from build123d import *

# Parameters (mm, degrees)
SKETCH1_W           = 203.2
SKETCH1_H           = 63.5
BOSS_EXTRUDE1_DEPTH = 3.175
SKETCH2_W           = 15.875
SKETCH2_H           = 6.35
CUT_EXTRUDE1_DEPTH  = 107.634633211
SKETCH3_W           = 19.05
SKETCH3_H           = 6.35
CUT_EXTRUDE2_DEPTH  = 107.634633211
LPATTERN1_COUNT     = 4
LPATTERN1_PITCH     = 38.1
SKETCH4_W           = 6.35
SKETCH4_H           = 19.05
CUT_EXTRUDE3_DEPTH  = 107.634633211


with BuildPart() as part:
    # Sketch1 → Boss-Extrude1 (new, symmetric)
    with BuildSketch(Plane.XY):
        Rectangle(SKETCH1_W, SKETCH1_H)
    extrude(amount=BOSS_EXTRUDE1_DEPTH, both=True)

    # Sketch2 → Cut-Extrude1 (cut, through all)
    with BuildSketch(Plane.XY.offset(3.175)):
        with Locations((-93.6625, 28.575)):
            Rectangle(SKETCH2_W, SKETCH2_H)
    cut_extrude1 = extrude(amount=-CUT_EXTRUDE1_DEPTH, mode=Mode.SUBTRACT)

    # Mirror1: Cut-Extrude1 across plane
    add(cut_extrude1.mirror(Plane(origin=(0, 0, 0), x_dir=(0, 0, 1), z_dir=(1, 0, 0))), mode=Mode.SUBTRACT)

    # Sketch3 → Cut-Extrude2 (cut, through all)
    with BuildSketch(Plane.XY.offset(3.175)):
        with Locations((-57.15, 28.575)):
            Rectangle(SKETCH3_W, SKETCH3_H)
    cut_extrude2 = extrude(amount=-CUT_EXTRUDE2_DEPTH, mode=Mode.SUBTRACT)

    # LPattern1: Cut-Extrude2 ×4
    with Locations(*[(i * LPATTERN1_PITCH, 0, 0) for i in range(1, LPATTERN1_COUNT)]):
        add(cut_extrude2, mode=Mode.SUBTRACT)

    # Sketch4 → Cut-Extrude3 (cut, through all)
    with BuildSketch(Plane.XY.offset(3.175)):
        with Locations((-98.425, 15.875)):
            Rectangle(SKETCH4_W, SKETCH4_H)
        with Locations((-98.425, -22.225)):
            Rectangle(SKETCH4_W, SKETCH4_H)
    cut_extrude3 = extrude(amount=-CUT_EXTRUDE3_DEPTH, mode=Mode.SUBTRACT)

    # Mirror2: Cut-Extrude3 across plane
    add(cut_extrude3.mirror(Plane(origin=(0, 0, 0), x_dir=(0, 0, 1), z_dir=(1, 0, 0))), mode=Mode.SUBTRACT)


solid = part.part
Geometry check sheet. Reference: the model listing, model coordinates, mm. A direction names the side the tool comes from. Round coordinates to 2 decimals unless told otherwise and drop trailing zeros. Write each loop counter-clockwise with the first axis right and the second up, starting at its lowest first coordinate (ties: lowest second). Pieces come first, ordered by that corner, then holes. Notation, with made-up numbers: (-27.5, -16.5) -> (23.5, -16.5) arc R22 ccw to (23.5, 4.5) -> close; hole circle Ø9 at (-33, 38). An arc over 180 degrees is marked (long way). One line per item, written item: value. Start each with the question number.
(1) Cross-section at B-B, the plane y = -21. Record the cut outline in (x, z) (3 decimals).
(2) Cross-section at C-C, the plane x = 54.5. Record the cut outline in (y, z) (3 decimals), and give its area (3 significant figures).
(3) Draft check along X on faces 5 (the flat face through (-101.6, -3, 0)), 6 (the flat face through (66.675, 29, 0)), 7 (the flat face through (-66.675, 29, 0)), 8 (the flat face through (95.25, -22, 0)). Enter one of: +X half, -X half, draft (parallel to the pull), parting line (faces both ways), or undercut.
(4) Scan lines: line 1 (X direction, y = 26.5, z = -0.5) (3 decimals); line 2 (X direction, y = -18.5, z = 0); line 3 (Y direction, x = 92.5, z = -1.5). Record each from-to range of solid material in increasing order. Write a range as [from, to].
(5) Access from +Z, -Z, +X, -X, +Y, -Y to the whole of each face (thin tool, end or side, straight path). Record for faces 1 (the flat face through (-95.25, 16, 0)), 2 (the flat face through (57, 25.4, 0)), 3 (the flat face through (-98, -12.7, 0)), 4 (the flat face through (95.25, 16, 0)).
(6) Go/stop test with flat-tipped pins: pin 1 Ø1.9 at (y, z) = (-23, 0.5) entering from -X; pin 2 Ø3 at (y, z) = (29, -1) entering from +X (3 decimals); pin 3 Ø3 at (x, z) = (89.5, -1.5) entering from +Y. Record where each tip stops, or that it passes through.
Answer:
1. outline: (-95.25, -3.175) -> (95.25, -3.175) -> (95.25, 3.175) -> (-95.25, 3.175) -> close
2. outline: (-31.75, -3.175) -> (25.4, -3.175) -> (25.4, 3.175) -> (-31.75, 3.175) -> close
2. area: 363 mm²
3. face 5: -X half
3. face 6: undercut
3. face 7: undercut
3. face 8: +X half
4. line 1: [-85.725, -66.675], [-47.625, -28.575], [-9.525, 9.525], [28.575, 47.625], [66.675, 85.725]
4. line 2: [-95.25, 95.25]
4. line 3: [-31.75, 25.4]
5. face 1: +Z, -Z, -X, +Y
5. face 2: +Z, -Z, +Y
5. face 3: +Z, -Z, -X, -Y
5. face 4: +Z, -Z, +X, +Y
6. pin 1: x = -95.25
6. pin 2: x = 85.725
6. pin 3: y = 25.4
